Autodesk Inventor part; units mm, degrees
ref_plane "Start Plane" through (0, 0, -50) normal (0, 0, 1) x (1, 0, 0)
ref_plane "End Plane" through (0, 0, 300) normal (0, 0, 1) x (1, 0, 0)
ref_plane "Work Plane5" through (0, -50, -50) normal (0, 0.7071, -0.7071) x (1, 0, 0)
ref_plane "Start Plane" through (0, 0, -50) normal (0, 0, 1) x (1, 0, 0)
ref_plane "End Plane" through (0, 0, 300) normal (0, 0, 1) x (1, 0, 0)
sketch "Sketch" plane through (0, 0, 0) normal (0, 0, 1) x (1, 0, 0)
  line L0 (-50, -44) -> (-50, 44)
  line L1 (-44, 50) -> (44, 50)
  line L2 (50, 44) -> (50, -44)
  line L3 (44, -50) -> (-44, -50)
  arc A0 (-50, -44) -> (-44, -50) centre (-44, -44) ccw
  arc A1 (50, 44) -> (44, 50) centre (44, 44) ccw
  arc A2 (-44, 50) -> (-50, 44) centre (-44, 44) ccw
  arc A3 (44, -50) -> (50, -44) centre (44, -44) ccw
  arc A4 (-44, 47) -> (-47, 44) centre (-44, 44) ccw
  line L4 (-44, 47) -> (44, 47)
  arc A5 (47, 44) -> (44, 47) centre (44, 44) ccw
  line L5 (47, 44) -> (47, -44)
  arc A6 (44, -47) -> (47, -44) centre (44, -44) ccw
  line L6 (44, -47) -> (-44, -47)
  arc A7 (-47, -44) -> (-44, -47) centre (-44, -44) ccw
  line L7 (-47, -44) -> (-47, 44)
  line L8 (0, 71.7397) -> (0, -71.7397) construction
  line L9 (-71.7397, 0) -> (71.7397, 0) construction
  dimension "d7" = 6
  dimension "d9" = 100
  dimension "d11" = 100
  dimension "d12" = 3
  dimension "d15" = 50
  dimension "d16" = 50
extrude "Body" add sketch "Sketch" along normal up to surface (350 mm away) from surface at -50
sketch "Sketch3" plane through (0, 0, 0) normal (0, 0, 1) x (1, 0, 0)
  line L0 (0, 0) -> (10, 0)
ref_plane "Work Plane3" through (0, 0, 0) normal (0, -1, 0) x (1, 0, 0)
sketch "Sketch5" plane through (44, 50, 300) normal (0, 1, 0) x (1, 0, 0)
  line L0 (3, 0) -> (3, 350)
  line L1 (-91, 350) -> (3, 350)
  line L2 (3, 350) -> (3, 250)
  line L3 (3, 250) -> (-91, 250)
  line L4 (-91, 250) -> (-91, 350)
  point P0 (-44, 300)
  point P1 (3, 300)
  point P2 (3, 300)
  dimension "d19" = 100
extrude "Extrusion2" cut sketch "Sketch5" against normal blind 10
ref_plane "Work Plane5" through (0, -50, -50) normal (0, 0.7071, -0.7071) x (1, 0, 0)
split "Split2" plane through (0, -50, -50) removes the side toward (0, 0.7071, -0.7071)
sketch "Sketch4" plane through (0, 0, 0) normal (0, -1, 0) x (1, 0, 0)
  line L0 (-2, -50) -> (12, -50)
  line L1 (-2, 300) -> (12, 300)
  dimension "d18" = 350
equation "\"d7\" = G_IR"
equation "\"d9\" = G_W"
equation "\"d11\" = G_H"
equation "\"d12\" = G_T"
equation "\"d15\" = 0.5 * d9"
equation "\"d16\" = 0.5 * d11"
equation "\"d3\" = G_L"
equation "\"G_W\" = 100"
equation "\"G_H\" = 100"
equation "\"G_T\" = 3"
equation "\"G_IR\" = 6"
equation "\"G_L\" = d18"
equation "\"G_OFFSET_END\" = 0"
properties part number "ISO 10799-2 - 100x100x3 - 350" material "Steel, Mild"
Model file for the job. Use its own axes, mm. A direction names the side the tool comes from. Give positions to 0.01 mm unless a question says otherwise; leave off trailing zeros. Write each loop counter-clockwise with the first axis right and the second up, starting at its lowest first coordinate (ties: lowest second). Pieces come first, ordered by that corner, then holes. Notation, with made-up numbers: (-28.5, 77.25) -> (0.5, 77.25) arc R34 cw to (0.5, 113.25) -> close; hole circle Ø9 at (65.5, -7.75). An arc over 180 degrees is marked (long way). Write item = value, one per line.
(1) Flat gauge pins, fed straight in: P1, Ø1.8, axis at x = -23, y = 46.5, coming from the -Z side; P2, Ø12, axis at x = 0.5, y = -36.5, coming from the -Z side. Where does each tip first touch, or does it go through?
Determined:
P1 = 50
P2 = through
(2) Slice it at C-C, the plane z = 101. Give the cut face in (x, y), then the cut area to 3 significant figures.
Determined:
outline = (-50, -44) arc R6 ccw to (-44, -50) -> (44, -50) arc R6 ccw to (50, -44) -> (50, 44) arc R6 ccw to (44, 50) -> (-44, 50) arc R6 ccw to (-50, 44) -> close; hole (-47, -44) arc R3 ccw to (-44, -47) -> (44, -47) arc R3 ccw to (47, -44) -> (47, 44) arc R3 ccw to (44, 47) -> (-44, 47) arc R3 ccw to (-47, 44) -> close
area = 1,140 mm2
(3) Slice it at A-A, the plane y = 9. Give the cut face in (x, z).
Determined:
outline = (-50, 9) -> (-47, 9) -> (-47, 300) -> (-50, 300) -> close; (47, 9) -> (50, 9) -> (50, 300) -> (47, 300) -> close
(4) Tool access for faces 4 (the face through (1, -47, 124)), 5 (the face through (-1, 50, 173)), 6 (the face through (1, 48, 50)): list every direction of +Z, -Z, +X, -X, +Y, -Y with a clear straight run to the whole face (end or side of a thin tool).
Determined:
face_4 = +Z, -Z
face_5 = +Z, -Z, +X, -X, +Y
face_6 = -Z, +Y
(5) Slice it at B-B, the plane x = -3.5. Give the cut face in (y, z).
Determined:
outline = (-50, -50) -> (-47, -47) -> (-47, 300) -> (-50, 300) -> close; (47, 50) -> (50, 50) -> (50, 300) -> (47, 300) -> close
(6) Mould opens along Y. For faces 1 (the face through (50, 1, 164)), 2 (the face through (48.196, 48.289, 170.208)), 3 (the face through (-47, -7, 130)) say: released by +Y, released by -Y, zero draft, split by the parting line, or undercut.
Determined:
face_1 = zero draft
face_2 = released by +Y
face_3 = undercut
(7) Probe line 1 along X through (y, z) = (-7, 155.5); line 2 along Y through (x, z) = (4, 17). List the from-to ranges inside material, lowest first.
Determined:
line_1 = -50 to -47, 47 to 50
line_2 = -50 to -47
